Here's how the part is built. I have some questions about the finished solid (model axes, mm). A direction names the side the tool comes from. Coordinates: 2 decimals unless noted, no trailing zeros. Loops run counter-clockwise (first coordinate to the right, second up) from the corner with the lowest first, then second, coordinate; pieces in that order, holes last.
from build123d import *

# Parameters (mm, degrees)
F1_DEPTH = 106.3625
F2_T     = -0.508


with BuildPart() as f1:
    # F0 (on Right) → F1 (new body, symmetric)
    with BuildSketch(Plane.YZ):
        with BuildLine():
            ThreePointArc((-218.7567022563, 6.35), (-152.3960137837, 63.4203756425), (-92.075, 0))
            Line((-92.075, 0), (0, 0))
            Line((0, 0), (99.695, 0))
            ThreePointArc((99.695, 0), (147.1808219158, 56.3269576842), (210.7265367264, 19.05))
            Line((210.7265367264, 19.05), (239.395, 9.525))
            Line((239.395, 9.525), (239.395, 88.9))
            Line((239.395, 88.9), (42.545, 88.9))
            Line((42.545, 88.9), (42.545, 158.75))
            Line((42.545, 158.75), (-71.755, 158.75))
            Line((-71.755, 158.75), (-93.98, 88.9))
            Line((-93.98, 88.9), (-243.205, 88.9))
            Line((-243.205, 88.9), (-243.205, 6.35))
            Line((-243.205, 6.35), (-218.7567022563, 6.35))
        make_face()
    extrude(amount=F1_DEPTH, both=True)

    # F2
    f2_openings = [f1.faces().sort_by_distance(p)[0] for p in [
        (0, 3.81, 0),
        (0, 147.180822, 56.326958),
        (0, 225.060768, 14.2875),
        (0, -152.396014, 63.420376),
        (0, -230.980851, 6.35),
    ]]
    offset(amount=F2_T, openings=f2_openings, kind=Kind.INTERSECTION)


solid = f1.part
Q1. For faces 1 (the flat face through (1, 42.545, 123)), 2 (the flat face through (1, 142, 88.392)), 3 (the cylindrical face through (106.112, -153.747, 63.474)), which set-ups out of +Z, -Z, +X, -X, +Y, -Y let a thin tool reach every point of the face, with its end or its side?
Q2. We'd pull the mould along X, two halves only. Please class faces 4 (the flat face through (0, -243, 6.35)), 5 (the flat face through (1, -14, 158.242)): pulls with the +X half, pulls with the -X half, needs draft (parallel to the pull), parting line crosses it, or undercut.
Q3. Suppose I cut it at D-D on z = 38.5. Write out the boundary of the cut face in (x, y) (1 decimal), and give its area (3 significant figures).
Q4. Suppose I cut it at C-C on y = -170. Write out the boundary of the cut face in (x, z).
Q5. Please list where these lines run through material, in increasing order: probe 1 along Y at (x, z) = (-11.5, 46) (3 decimals); probe 2 along X at (y, z) = (101, 24); probe 3 along Y at (x, z) = (-5, 8.5) (3 decimals).
Q6. Suppose I cut it at B-B on x = 77.5. Write out the boundary of the cut face in (y, z) (3 decimals), and give its area (3 significant figures).
Q7. Will these pins go through, and if not, where does the flat tip stop? P1, Ø8, axis at x = 53, z = 89.5, coming from the +Y side (3 decimals); P2, Ø21, axis at x = -27.5, z = 137.5, coming from the -Y side; P3, Ø10, axis at x = -58, y = -6, coming from the -Z side; P4, Ø1, axis at x = -35, z = 125.5, coming from the -Y side.
Q8. Suppose I cut it at A-A on z = 76.5. Write out the boundary of the cut face in (x, y) (1 decimal), and give its area (3 significant figures).
Check values:
1. face 1: +Z, +X, -X, +Y
1. face 2: -Z
1. face 3: -Z, +X, -X
2. face 4: needs draft
2. face 5: undercut
3. outline: (-106.4, -243.2) - (106.4, -243.2) - (106.4, -206.1) - (105.9, -206.1) - (105.9, -242.7) - (-105.9, -242.7) - (-105.9, -206.1) - (-106.4, -206.1) - close; (-106.4, -105.1) - (-105.9, -105.1) - (-105.9, 114.6) - (-106.4, 114.6) - close; (-106.4, 199.1) - (-105.9, 199.1) - (-105.9, 238.9) - (105.9, 238.9) - (105.9, 199.1) - (106.4, 199.1) - (106.4, 239.4) - (-106.4, 239.4) - close; (105.9, -105.1) - (106.4, -105.1) - (106.4, 114.6) - (105.9, 114.6) - close
3. area: 517 mm2
4. outline: (-106.36, 61.84) - (-105.85, 61.84) - (-105.85, 88.39) - (105.85, 88.39) - (105.85, 61.84) - (106.36, 61.84) - (106.36, 88.9) - (-106.36, 88.9) - close
5. probe 1: y = -243.205 to -242.697, 238.887 to 239.395
5. probe 2: x = -106.36 to -105.85, 105.85 to 106.36
5. probe 3: y = -243.205 to -242.697
6. outline: (-243.205, 6.35) - (-242.697, 6.35) - (-242.697, 88.392) - (-93.609, 88.392) - (-71.384, 158.242) - (42.037, 158.242) - (42.037, 88.392) - (238.887, 88.392) - (238.887, 9.694) - (239.395, 9.525) - (239.395, 88.9) - (42.545, 88.9) - (42.545, 158.75) - (-71.755, 158.75) - (-93.98, 88.9) - (-243.205, 88.9) - close
6. area: 388 mm2
7. P1: stops at y = 239.395
7. P2: stops at y = -81.86
7. P3: stops at z = 158.24
7. P4: stops at y = -82.49
8. outline: (-106.4, -243.2) - (106.4, -243.2) - (106.4, 239.4) - (-106.4, 239.4) - close; hole (-105.9, -242.7) - (105.9, -242.7) - (105.9, 238.9) - (-105.9, 238.9) - close
8. area: 705 mm2
